```python
from build123d import *

# Parameters (mm, degrees)
SKETCH_1_W               = 46.3
SKETCH_1_H               = 12
EXTRUDE_1_DEPTH          = 3.5
SKETCH_2_W               = 3
SKETCH_2_H               = 12
EXTRUDE_2_DEPTH          = 6
CUT_EXTRUDE_1_DEPTH      = 45.734103322
CUT_EXTRUDE_1_DEPTH_BACK = 45.734103322
SKETCH_3_R               = 1.65
CHAMFER_1_SIZE           = 2
CHAMFER_2_SIZE           = 2
CUT_EXTRUDE_2_DEPTH      = 25.656084442
CUT_EXTRUDE_2_DEPTH_BACK = 25.656084442
FILLET_1_R               = 0.2


with BuildPart() as part:
    # 草图1 → 凸台-拉伸1 (new body)
    with BuildSketch(Plane.XY):
        Rectangle(SKETCH_1_W, SKETCH_1_H)
    extrude(amount=EXTRUDE_1_DEPTH)

    # 草图2 → 凸台-拉伸2 (add)
    with BuildSketch(Plane.XY.offset(3.5)):
        with Locations((-21.65, 0)):
            Rectangle(SKETCH_2_W, SKETCH_2_H)
        with Locations((21.65, 0)):
            Rectangle(SKETCH_2_W, SKETCH_2_H)
    extrude(amount=EXTRUDE_2_DEPTH)

    # 草图3 → 切除-拉伸1 (cut, two sides: drawn at the far end of the back side and taken through both)
    with BuildSketch(Plane(origin=(-20.15, 0, 0), x_dir=(0, 0, -1), z_dir=(1, 0, 0)).offset(-CUT_EXTRUDE_1_DEPTH_BACK)):
        with Locations((-6.5, 0.001559283)):
            Circle(SKETCH_3_R)
    extrude(amount=CUT_EXTRUDE_1_DEPTH + CUT_EXTRUDE_1_DEPTH_BACK, mode=Mode.SUBTRACT)

    # 倒角1
    chamfer_1_edges = [part.edges().sort_by_distance(p)[0] for p in [
        (-23.15, 0, 0),
        (23.15, 0, 0),
    ]]
    chamfer(chamfer_1_edges, length=CHAMFER_1_SIZE)

    # 倒角2
    chamfer_2_edges = [part.edges().sort_by_distance(p)[0] for p in [
        (-21.65, -6, 9.5),
        (-21.65, 6, 9.5),
        (21.65, 6, 9.5),
        (21.65, -6, 9.5),
    ]]
    chamfer(chamfer_2_edges, length=CHAMFER_2_SIZE)

    # 草图4 → 切除-拉伸2 (cut, two sides: drawn at the far end of the back side and taken through both)
    with BuildSketch(Plane.XY.offset(3.5).offset(-CUT_EXTRUDE_2_DEPTH_BACK)):
        Polygon((-8.177250548, 4), (8.177250548, 4), (0, 1.565086686), align=None)
        Polygon((-16.15, 3.243846317), (-16.15, -3.243846317), (-5.256082786, 0), align=None)
        Polygon((8.177250548, -4), (0, -1.565086686), (-8.177250548, -4), align=None)
        Polygon((16.15, -3.243846317), (5.256082786, 0), (16.15, 3.243846317), align=None)
    extrude(amount=CUT_EXTRUDE_2_DEPTH + CUT_EXTRUDE_2_DEPTH_BACK, mode=Mode.SUBTRACT)

    # 圆角1
    fillet_1_edges = [part.edges().sort_by_distance(p)[0] for p in [
        (-8.177250548, 4, 1.75),
        (8.177250548, 4, 1.75),
        (8.177250548, -4, 1.75),
        (-8.177250548, -4, 1.75),
        (16.15, 3.243846317, 1.75),
        (16.15, -3.243846317, 1.75),
        (5.256082786, 0, 1.75),
        (-16.15, 3.243846317, 1.75),
        (-5.256082786, 0, 1.75),
        (-16.15, -3.243846317, 1.75),
    ]]
    fillet(fillet_1_edges, radius=FILLET_1_R)


solid = part.part
```
For this review, take the finished solid that the model builds, in its own axes (mm). A direction names the side the tool comes from. Give positions to 0.01 mm unless a question says otherwise; leave off trailing zeros. Order: outer loops, then holes, each group sorted by start corner. A loop starts at its lowest first (then second) coordinate and runs counter-clockwise, first axis right, second up.
1) Take a section at B-B (z = 4). Give the boundary of the cut face in (x, y).
2) The part is to be moulded in two halves that separate along X. For faces 1 (the face through (23.15, 1, 5)), 2 (the face through (3.48, -2.6, 1.73)), 3 (the face through (21.63, 0.07, 8.15)), 4 (the face through (-22.14, -0.08, 0.99)), say which applies: released by +X, released by -X, zero draft, split by the parting line, or undercut.
3) For faces 5 (the face through (-3.38, 2.57, 1.73)), 6 (the face through (21.6, 5, 8.5)), 7 (the face through (20.15, 1, 5)), list the 3-axis set-ups (+Z, -Z, +X, -X, +Y, -Y) from which the entire face can be reached by the end or side of a thin tool; tool diameter is ignored.
4) Take a section at D-D (x = 9). Give the boundary of the cut face in (y, z), then the cut area to 3 significant figures.
5) Take a section at A-A (z = 6.5). Give the boundary of the cut face in (x, y), then the cut area to 3 significant figures.
6) Take a section at C-C (z = 0.5). Give the boundary of the cut face in (x, y).
7) Wall thickness on line 1 (X direction, y = 3, z = 9.25); line 2 (Y direction, x = 21.8, z = 6.5): over which ranges is each line inside the solid? List them lowest first.
8) Insertion check: pin 1 (3.5 mm diameter, centred on x = -9.5, y = -0.5, fed in from +Z). The pin has a flat end and moves straight along its axis. Give the tip position at first contact, or say it passes through.
Derived:
1. outline: (-23.15, -6) - (-20.15, -6) - (-20.15, 6) - (-23.15, 6) - close; (20.15, -6) - (23.15, -6) - (23.15, 6) - (20.15, 6) - close
2. face 1: released by +X
2. face 2: undercut
2. face 3: zero draft
2. face 4: released by -X
3. face 5: +Z, -Z
3. face 6: +Z, +X, -X, +Y
3. face 7: +Z, +Y, -Y
4. outline: (-6, 0) - (-1.11, 0) - (-1.11, 3.5) - (-6, 3.5) - close; (1.11, 0) - (6, 0) - (6, 3.5) - (1.11, 3.5) - close
4. area: 34.2 mm2
5. outline: (-23.15, -6) - (-20.15, -6) - (-20.15, -1.65) - (-23.15, -1.65) - close; (-23.15, 1.65) - (-20.15, 1.65) - (-20.15, 6) - (-23.15, 6) - close; (20.15, -6) - (23.15, -6) - (23.15, -1.65) - (20.15, -1.65) - close; (20.15, 1.65) - (23.15, 1.65) - (23.15, 6) - (20.15, 6) - close
5. area: 52.2 mm2
6. outline: (-21.65, -6) - (21.65, -6) - (21.65, 6) - (-21.65, 6) - close; hole (-16.15, -2.98) arc R0.2 ccw to (-15.89, -3.17) - (-5.9, -0.19) arc R0.2 ccw to (-5.9, 0.19) - (-15.89, 3.17) arc R0.2 ccw to (-16.15, 2.98) - close; hole (-6.86, -3.61) arc R0.2 ccw to (-6.8, -4) - (6.8, -4) arc R0.2 ccw to (6.86, -3.61) - (0, -1.57) - close; hole (-6.86, 3.61) - (0, 1.57) - (6.86, 3.61) arc R0.2 ccw to (6.8, 4) - (-6.8, 4) arc R0.2 ccw to start; hole (5.9, -0.19) - (15.89, -3.17) arc R0.2 ccw to (16.15, -2.98) - (16.15, 2.98) arc R0.2 ccw to (15.89, 3.17) - (5.9, 0.19) arc R0.2 ccw to start
7. line 1: x = -23.15 to -20.15, 20.15 to 23.15
7. line 2: y = -6 to -1.65, 1.65 to 6
8. pin 1: stops at z = 3.5
